Answer from the drawing. Dimensions are ordinates in mm from the lowest x, y and z of the part. A direction names the side the tool comes from. Coordinates: 2 decimals unless noted, no trailing zeros. Order: outer loops, then holes, each group sorted by start corner. A loop starts at its lowest first (then second) coordinate and runs counter-clockwise, first axis right, second up. Notation, with made-up numbers: (-35, 48.5) - (-4, 48.5) arc R24 cw to (-4, 66.5) - close; hole circle Ø11 at (57, 52.5). An arc over 180 degrees is marked (long way). Use a Markdown table: item, result. Add a question column.
Item 1: The part is cut by section A-A, the plane x = 24. Give the vertices of the cut face in (y, z), then the cut area to 3 significant figures.
Item 2: The part is cut by section C-C, the plane y = 33.47. Give the vertices of the cut face in (x, z).
Item 3: Find the intervals of material crossed by line 1 along Z through (x, y) = (19.5, 33.47); line 2 along Y through (x, z) = (8.25, 62.39); line 3 along X through (y, z) = (7, 70.5), in increasing order.
Item 4: The mould has two halves that part along Z. Classify the marked faces 4, 5 and 6: released by +Z, released by -Z, zero draft, split by the parting line, or undercut.
Item 5: For the marked faces 1, 2 and 3, determine the directions among +Z, -Z, +X, -X, +Y, -Y from which every point of the face is accessible in a straight line to the end or side of a thin tool.
Item 6: The part is cut by section B-B, the plane z = 62.39. Give the vertices of the cut face in (x, y).
Item 7: The part is cut by section D-D, the plane x = 6. Give the vertices of the cut face in (y, z).
Item 8: Flat-ended cylindrical pins translate along their axes: P1, Ø1.5, axis at x = 7.5, z = 10, coming from the -Y side; P2, Ø10, axis at x = 9, y = 20.5, coming from the +Z side; P3, Ø8.5, axis at y = 30.5, z = 51, coming from the -X side; P4, Ø14.5, axis at y = 24, z = 24, coming from the +X side. Find the tip coordinate at first contact, or state that the pin passes through.
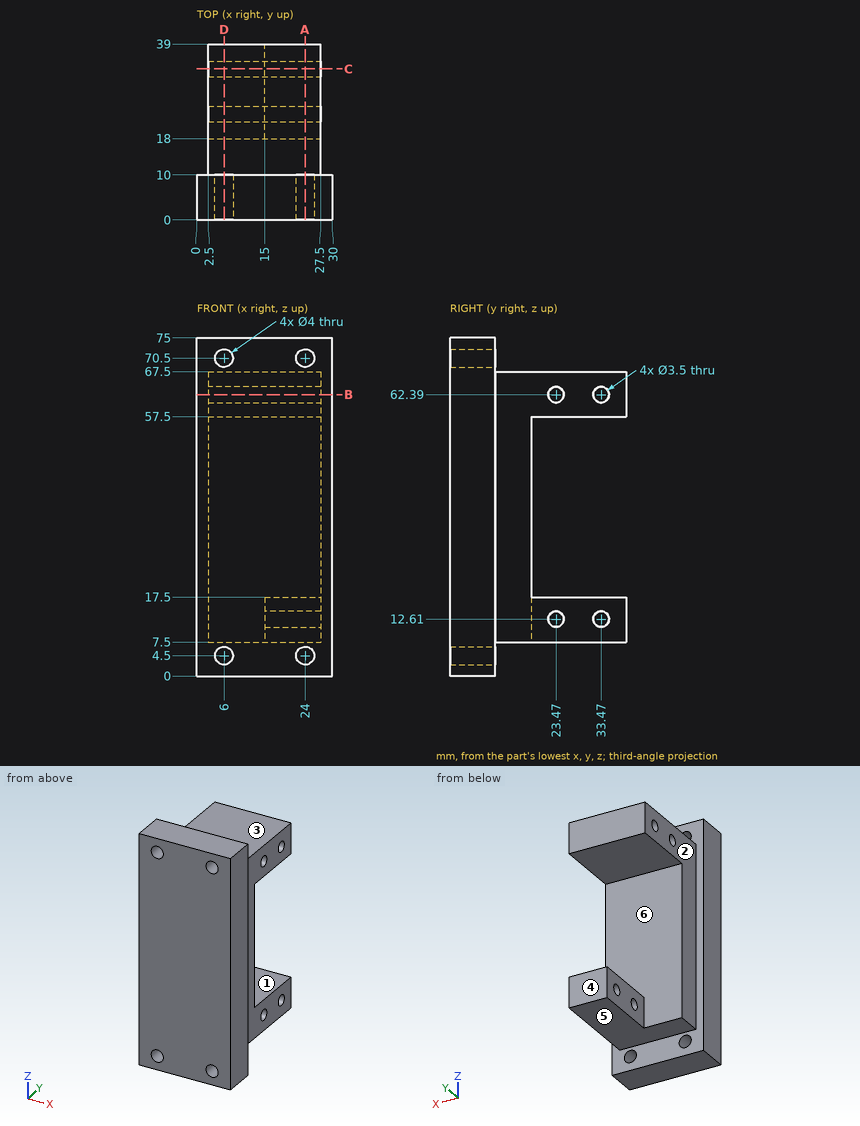
Solution:
| question | item | result |
|---|---|---|
| 1 | outline | (0, 0) - (10, 0) - (10, 2.5) - (0, 2.5) - close; (0, 6.5) - (10, 6.5) - (10, 7.5) - (39, 7.5) - (39, 17.5) - (18, 17.5) - (18, 57.5) - (39, 57.5) - (39, 67.5) - (10, 67.5) - (10, 68.5) - (0, 68.5) - close; (0, 72.5) - (10, 72.5) - (10, 75) - (0, 75) - close; hole circle Ø3.5 at (23.47, 12.61); hole circle Ø3.5 at (23.47, 62.39); hole circle Ø3.5 at (33.47, 12.61); hole circle Ø3.5 at (33.47, 62.39) |
| 1 | area | 1,530 mm2 |
| 2 | outline | (2.5, 57.5) - (27.5, 57.5) - (27.5, 60.64) - (2.5, 60.64) - close; (2.5, 64.14) - (27.5, 64.14) - (27.5, 67.5) - (2.5, 67.5) - close; (15, 7.5) - (27.5, 7.5) - (27.5, 10.86) - (15, 10.86) - close; (15, 14.36) - (27.5, 14.36) - (27.5, 17.5) - (15, 17.5) - close |
| 3 | line 1 | z = 7.5 to 10.86, 14.36 to 17.5, 57.5 to 60.64, 64.14 to 67.5 |
| 3 | line 2 | y = 0 to 21.72, 25.22 to 31.72, 35.22 to 39 |
| 3 | line 3 | x = 0 to 4, 8 to 22, 26 to 30 |
| 4 | face 4 | zero draft |
| 4 | face 5 | released by -Z |
| 4 | face 6 | undercut |
| 5 | face 1 | +X, -X, +Y |
| 5 | face 2 | +Z, -Z, -X, +Y |
| 5 | face 3 | +Z, +X, -X, +Y |
| 6 | outline | (0, 0) - (30, 0) - (30, 10) - (27.5, 10) - (27.5, 21.72) - (2.5, 21.72) - (2.5, 10) - (0, 10) - close; (2.5, 25.22) - (27.5, 25.22) - (27.5, 31.72) - (2.5, 31.72) - close; (2.5, 35.22) - (27.5, 35.22) - (27.5, 39) - (2.5, 39) - close |
| 7 | outline | (0, 0) - (10, 0) - (10, 2.5) - (0, 2.5) - close; (0, 6.5) - (10, 6.5) - (10, 7.5) - (18, 7.5) - (18, 57.5) - (39, 57.5) - (39, 67.5) - (10, 67.5) - (10, 68.5) - (0, 68.5) - close; (0, 72.5) - (10, 72.5) - (10, 75) - (0, 75) - close; hole circle Ø3.5 at (23.47, 62.39); hole circle Ø3.5 at (33.47, 62.39) |
| 8 | P1 | stops at y = 0 |
| 8 | P2 | stops at z = 67.5 |
| 8 | P3 | passes through |
| 8 | P4 | stops at x = 27.5 |
